Design review of the part built by this model. Coordinates are the model's own, in mm. A direction names the side the tool comes from. Give positions to 0.01 mm unless a question says otherwise; leave off trailing zeros. Write each loop counter-clockwise with the first axis right and the second up, starting at its lowest first coordinate (ties: lowest second). Pieces come first, ordered by that corner, then holes.
```python
from build123d import *

# Parameters (mm, degrees)
SKETCH_1_R          = 4
EXTRUDE_1_DEPTH     = 12.5
SKETCH_2_W          = 25.15
SKETCH_2_H          = 5
CUT_EXTRUDE_1_DEPTH = 16


with BuildPart() as part:
    # 草图1 → 凸台-拉伸1 (new, symmetric)
    with BuildSketch(Plane(origin=(0, 0, 0), x_dir=(1, 0, 0), z_dir=(0, 1, 0))):
        with BuildLine():
            Line((0, 8), (29.228297239, 8))
            Line((29.228297239, 8), (48.144548452, 57.11524489))
            ThreePointArc((48.144548452, 57.11524489), (58.48524489, 61.705451548), (63.075451548, 51.36475511))
            Line((63.075451548, 51.36475511), (42.185451548, -2.87524489))
            ThreePointArc((42.185451548, -2.87524489), (39.247584393, -6.595527239), (34.72, -8))
            Line((34.72, -8), (0, -8))
            ThreePointArc((0, -8), (-8, 0), (0, 8))
        make_face()
        with Locations(Location((0, 0, 0), (0, 0, 270))):
            Circle(SKETCH_1_R, mode=Mode.SUBTRACT)
        with Locations(Location((34.72, 0, 0), (0, 0, 270))):
            Circle(SKETCH_1_R, mode=Mode.SUBTRACT)
        with Locations(Location((55.61, 54.24, 0), (0, 0, 270))):
            Circle(SKETCH_1_R, mode=Mode.SUBTRACT)
    extrude(amount=EXTRUDE_1_DEPTH, both=True)

    # 草图2 → 切除-拉伸1 (cut)
    with BuildSketch(Plane.XY.offset(8)):
        with Locations((4.575, 0)):
            Rectangle(SKETCH_2_W, SKETCH_2_H)
    extrude(amount=-CUT_EXTRUDE_1_DEPTH, mode=Mode.SUBTRACT)


solid = part.part
```
(1) Clearance check with flat-ended pins moving along their axes: P1, Ø7, axis at x = 0, z = 0, coming from the -Y side; P2, Ø2, axis at x = 47.5, y = -8, coming from the -Z side; P3, Ø5, axis at y = 6, z = -16, coming from the +X side; P4, Ø2, axis at y = 3, z = -24.5, coming from the -X side. State where each tip first meets the part, or that it passes through.
Resolved:
P1: passes through
P2: stops at z = -57.91
P3: stops at x = 50.42
P4: stops at x = 35.2
(2) Consider section C-C, the plane y = 8.5. Give the boundary of the cut face in (x, z), then the cut area to 3 significant figures.
Resolved:
outline: (0, -8) - (29.23, -8) - (48.14, -57.12) arc R8 ccw to (63.08, -51.36) - (42.19, 2.88) arc R8 ccw to (34.72, 8) - (0, 8) arc R8 ccw to start; hole circle Ø8 at (0, 0); hole circle Ø8 at (34.72, 0); hole circle Ø8 at (55.61, -54.24)
area: 1,530 mm2
(3) Consider section D-D, the plane z = -0.5. Give the boundary of the cut face in (x, y).
Resolved:
outline: (-7.98, -12.5) - (-3.97, -12.5) - (-3.97, -2.5) - (-7.98, -2.5) - close; (-7.98, 2.5) - (-3.97, 2.5) - (-3.97, 12.5) - (-7.98, 12.5) - close; (3.97, -12.5) - (30.75, -12.5) - (30.75, 12.5) - (3.97, 12.5) - (3.97, 2.5) - (17.15, 2.5) - (17.15, -2.5) - (3.97, -2.5) - close; (38.69, -12.5) - (43.49, -12.5) - (43.49, 12.5) - (38.69, 12.5) - close
(4) Tool access review of faces 4 (the face through (14, 3, -8)), 5 (the face through (17.15, 0, 0)), 6 (the face through (-8, 8, 0)): name each direction out of +Z, -Z, +X, -X, +Y, -Y from which nothing blocks a thin tool from reaching the whole face with its end or side.
Resolved:
face 4: -Z, -X, +Y, -Y
face 5: +Z, -Z, -X
face 6: -X, +Y, -Y
(5) Consider section B-B, the plane x = 32.5. Give the boundary of the cut face in (y, z).
Resolved:
outline: (-12.5, -16.49) - (12.5, -16.49) - (12.5, -3.33) - (-12.5, -3.33) - close; (-12.5, 3.33) - (12.5, 3.33) - (12.5, 8) - (-12.5, 8) - close
(6) Consider section A-A, the plane z = -54.24. Give the boundary of the cut face in (x, y).
Resolved:
outline: (47.04, -12.5) - (51.61, -12.5) - (51.61, 12.5) - (47.04, 12.5) - close; (59.61, -12.5) - (63.61, -12.5) - (63.61, 12.5) - (59.61, 12.5) - close
(7) Mouldability with a two-part tool opening along Z and no side actions: class faces 1 (the face through (30.815, -0.175, -0.867)), 2 (the face through (39.3, 0.18, 6.56)), 3 (the face through (33, -12.5, -17)) as pulls with the +Z half, pulls with the -Z half, needs draft (parallel to the pull), parting line crosses it, or undercut.
Resolved:
face 1: undercut
face 2: pulls with the +Z half
face 3: needs draft
(8) To check wall thickness, follow L1, parallel to Y at x = 1, z = -4; L2, parallel to X at y = -7.5, z = -2; L3, parallel to Z at x = 0, y = -5.75. State the ranges of each line that lie inside material, in increasing order.
Resolved:
L1: y = -12.5 to -2.5, 2.5 to 12.5
L2: x = -7.75 to -3.46, 3.46 to 31.26, 38.18 to 44.06
L3: z = -8 to -4, 4 to 8
